from build123d import *

# Parameters (mm, degrees)
F0_W     = 60
F0_H     = 60
F0_R     = 3.25
F1_DEPTH = 8
F0_R_2   = 1.5
F2_DEPTH = 13
F3_DEPTH = 5


with BuildPart() as f1:
    # F0 (on Top) → F1 (new body)
    with BuildSketch(Plane.XY):
        Rectangle(F0_W, F0_H)
        with Locations((-21.85, -21.85)):
            Circle(F0_R, mode=Mode.SUBTRACT)
        with Locations((21.85, -21.85)):
            Circle(F0_R, mode=Mode.SUBTRACT)
        with Locations((-21.85, 21.85)):
            Circle(F0_R, mode=Mode.SUBTRACT)
        with Locations((21.85, 21.85)):
            Circle(F0_R, mode=Mode.SUBTRACT)
    extrude(amount=F1_DEPTH)

    # F0 (on Top) → F2 (join)
    with BuildSketch(Plane.XY):
        with Locations((-21.85, 21.85)):
            Circle(F0_R)
        with Locations((-21.85, 21.85)):
            Circle(F0_R_2, mode=Mode.SUBTRACT)
        with Locations((21.85, 21.85)):
            Circle(F0_R)
        with Locations((21.85, 21.85)):
            Circle(F0_R_2, mode=Mode.SUBTRACT)
        with Locations((-21.85, -21.85)):
            Circle(F0_R)
        with Locations((-21.85, -21.85)):
            Circle(F0_R_2, mode=Mode.SUBTRACT)
        with Locations((21.85, -21.85)):
            Circle(F0_R)
        with Locations((21.85, -21.85)):
            Circle(F0_R_2, mode=Mode.SUBTRACT)
    extrude(amount=F2_DEPTH)

    # F0 (on Top) → F3 (join)
    with BuildSketch(Plane.XY):
        with Locations((-21.85, 21.85)):
            Circle(F0_R_2)
        with Locations((21.85, 21.85)):
            Circle(F0_R_2)
        with Locations((-21.85, -21.85)):
            Circle(F0_R_2)
        with Locations((21.85, -21.85)):
            Circle(F0_R_2)
    extrude(amount=F3_DEPTH)


solid = f1.part
Verification items for the finished model (mm, model axes). A direction names the side the tool comes from. Coordinates: 2 decimals unless noted, no trailing zeros. Write each loop counter-clockwise with the first axis right and the second up, starting at its lowest first coordinate (ties: lowest second). Pieces come first, ordered by that corner, then holes. Notation, with made-up numbers: (13, -17) -> (41, -17) arc R36 cw to (41, 22) -> close; hole circle Ø6 at (60, -19.75). An arc over 180 degrees is marked (long way). One line per item, written item: value. Start each with the question number.
Q1. Cross-section at A-A on z = 9. Enter the section's corners in (x, y), and give its area (3 significant figures).
Q2. Mould release check, pull along X, two halves, no side actions. Record for faces 3 (the flat face through (30, 0, 4)), 4 (the flat face through (-20, -23, 13)), 5 (the flat face through (22, 22, 5)): pulls with the +X half, pulls with the -X half, needs draft (parallel to the pull), parting line crosses it, or undercut.
Q3. Access from +Z, -Z, +X, -X, +Y, -Y to the whole of each face (thin tool, end or side, straight path). Record for faces 1 (the flat face through (0, 30, 4)), 2 (the cylindrical face through (23.35, -24.733, 10.465)).
Q4. Cross-section at D-D on y = -10. Enter the section's corners in (x, z), and give its area (3 significant figures).
Q5. Cross-section at B-B on x = -21.85. Enter the section's corners in (y, z).
Q6. Go/stop test with flat-tipped pins: P1, Ø8, axis at x = -11, y = 14.5, coming from the +Z side; P2, Ø1.5, axis at x = 22, y = 22, coming from the +Z side; P3, Ø2, axis at y = -3, z = 10.5, coming from the -X side. Record where each tip stops, or that it passes through.
Q7. Thickness scan on L1, parallel to Y at x = 21.85, z = 7.5; L2, parallel to Y at x = -21.85, z = 11.25; L3, parallel to X at y = 21, z = 12. Record the ranges inside material, lowest first. Write a range as from..to.
Checked values:
1. outline: circle Ø6.5 at (-21.85, -21.85); circle Ø6.5 at (-21.85, 21.85); circle Ø6.5 at (21.85, -21.85); circle Ø6.5 at (21.85, 21.85); hole circle Ø3 at (-21.85, -21.85); hole circle Ø3 at (-21.85, 21.85); hole circle Ø3 at (21.85, -21.85); hole circle Ø3 at (21.85, 21.85)
1. area: 104 mm²
2. face 3: pulls with the +X half
2. face 4: needs draft
2. face 5: undercut
3. face 1: +Z, -Z, +X, -X, +Y
3. face 2: +Z
4. outline: (-30, 0) -> (30, 0) -> (30, 8) -> (-30, 8) -> close
4. area: 480 mm²
5. outline: (-30, 0) -> (30, 0) -> (30, 8) -> (25.1, 8) -> (25.1, 13) -> (23.35, 13) -> (23.35, 5) -> (20.35, 5) -> (20.35, 13) -> (18.6, 13) -> (18.6, 8) -> (-18.6, 8) -> (-18.6, 13) -> (-20.35, 13) -> (-20.35, 5) -> (-23.35, 5) -> (-23.35, 13) -> (-25.1, 13) -> (-25.1, 8) -> (-30, 8) -> close
6. P1: stops at z = 8
6. P2: stops at z = 5
6. P3: passes through
7. L1: y = -30..-23.35, -20.35..20.35, 23.35..30
7. L2: y = -25.1..-23.35, -20.35..-18.6, 18.6..20.35, 23.35..25.1
7. L3: x = -24.99..-23.09, -20.61..-18.71, 18.71..20.61, 23.09..24.99
